```python
from build123d import *

# Parameters (mm, degrees)
BOSS_EXTRUDE1_DEPTH     = 100
BOSS_EXTRUDE1_TAPER     = 18.43
SKETCH2_W               = 170
SKETCH2_H               = 190
BOSS_EXTRUDE2_DEPTH     = 90
SKETCH3_R               = 1.35
BOSS_EXTRUDE3_DEPTH     = 10
SKETCH4_W               = 180
SKETCH4_H               = 50
CUT_EXTRUDE1_DEPTH      = 286.000000111
SKETCH5_R               = 2.5
CUT_EXTRUDE2_DEPTH      = 10
SKETCH6_R               = 8
CUT_EXTRUDE3_DEPTH      = 10
MIRROR4_COPY_1_SKETCH_R = 8
MIRROR4_COPY_1_DEPTH    = 10


with BuildPart() as part:
    # Sketch1 → Boss-Extrude1 (new body)
    with BuildSketch(Plane(origin=(0, 0, 0), x_dir=(1, 0, 0), z_dir=(0, 1, 0))):
        Polygon((-140, -45), (-125, -60), (-95, -90), (95, -90), (140, -45), (140, 45), (95, 90), (-95, 90), (-140, 45), align=None)
    extrude(amount=BOSS_EXTRUDE1_DEPTH, taper=BOSS_EXTRUDE1_TAPER)

    # Sketch2 → Boss-Extrude2 (add, symmetric)
    with BuildSketch(Plane.XY):
        with Locations((0, 45)):
            Rectangle(SKETCH2_W, SKETCH2_H)
    extrude(amount=BOSS_EXTRUDE2_DEPTH, both=True)

    # Sketch3 → Boss-Extrude3 (add, symmetric)
    with BuildSketch(Plane(origin=(0, 140, 0), x_dir=(1, 0, 0), z_dir=(0, 1, 0))):
        with Locations(Location((-70, 87.5, 0), (0, 0, 90))):
            Circle(SKETCH3_R)
        with Locations(Location((70, 87.5, 0), (0, 0, 90))):
            Circle(SKETCH3_R)
    boss_extrude3 = extrude(amount=BOSS_EXTRUDE3_DEPTH, both=True)

    # Mirror1: Boss-Extrude3 across plane
    add(boss_extrude3.mirror(Plane.XY))

    # Sketch4 → Cut-Extrude1 (cut, through all)
    with BuildSketch(Plane.ZY.offset(85)):
        with Locations((0, -25)):
            Rectangle(SKETCH4_W, SKETCH4_H)
    extrude(amount=-CUT_EXTRUDE1_DEPTH, mode=Mode.SUBTRACT)

    # Sketch5 → Cut-Extrude2 (cut)
    with BuildSketch(Plane(origin=(0, 0, -90), x_dir=(-1, 0, 0), z_dir=(0, 0, -1))):
        with Locations((-60, 133)):
            Circle(SKETCH5_R)
        with Locations((60, 133)):
            Circle(SKETCH5_R)
    cut_extrude2 = extrude(amount=-CUT_EXTRUDE2_DEPTH, mode=Mode.SUBTRACT)

    # Mirror2: Cut-Extrude2 across plane
    add(cut_extrude2.mirror(Plane.XY), mode=Mode.SUBTRACT)

    # Sketch6 → Cut-Extrude3 (cut)
    with BuildSketch(Plane(origin=(-83.254793164, 39.235386654, -83.254793164), x_dir=(-0.6068291050905237, 0.2859796255102721, 0.741602380665029), z_dir=(-0.6708397043943968, 0.31614582397380636, -0.6708397043943966))):
        with Locations(Location((23.427974197, -19.317213572, 0), (0, 0, 342.455867608))):
            Circle(SKETCH6_R)
        with Locations(Location((47.265100386, -26.853221472, 0), (0, 0, 342.455867608))):
            Circle(SKETCH6_R)
    cut_extrude3 = extrude(amount=-CUT_EXTRUDE3_DEPTH, mode=Mode.SUBTRACT)

    # Mirror3: Cut-Extrude3 across plane
    add(cut_extrude3.mirror(Plane.XY), mode=Mode.SUBTRACT)

    # Mirror4: Cut-Extrude3 across plane
    add(cut_extrude3.mirror(Plane(origin=(0, 0, 0), x_dir=(0, 0, 1), z_dir=(1, 0, 0))), mode=Mode.SUBTRACT)

    # Mirror4 copy 1 sketch → Mirror4 copy 1 (cut)
    with BuildSketch(Plane(origin=(83.254793164, 39.235386654, 83.254793164), x_dir=(0.6068291050905237, 0.2859796255102721, -0.741602380665029), z_dir=(0.6708397043943968, 0.31614582397380636, 0.6708397043943966))):
        with Locations(Location((23.427974197, -19.317213572, 0), (0, 0, 342.455867608))):
            Circle(MIRROR4_COPY_1_SKETCH_R)
        with Locations(Location((47.265100386, -26.853221472, 0), (0, 0, 342.455867608))):
            Circle(MIRROR4_COPY_1_SKETCH_R)
    extrude(amount=-MIRROR4_COPY_1_DEPTH, mode=Mode.SUBTRACT)


solid = part.part
```
Verification items for the finished model (mm, model axes). A direction names the side the tool comes from. Give positions to 0.01 mm unless a question says otherwise; leave off trailing zeros. Order: outer loops, then holes, each group sorted by start corner. A loop starts at its lowest first (then second) coordinate and runs counter-clockwise, first axis right, second up. Notation, with made-up numbers: M 10,-39.75 L 55,-39.75 A14 ccw 55,-12.75 Z; hole C -3.75,-0.5 d7. An arc over 180 degrees is marked long. Return JSON: item names as keys, results as strings. Group by question number.
1) Section check B-B on y = 118. Record the cut outline in (x, z), and give its area (3 significant figures).
2) Access from +Z, -Z, +X, -X, +Y, -Y to the whole of each face (thin tool, end or side, straight path). Record for faces 4 (the face through (-1, 71, 90)), 5 (the face through (-92, 100, 3)), 6 (the face through (-116.57, 25.41, -41.55)).
3) Go/stop test with flat-tipped pins: pin 1 Ø11 at (x, z) = (92.5, 20) entering from +Y; pin 2 Ø1.5 at (x, y) = (-59.5, 133) entering from +Z; pin 3 Ø1.5 at (y, z) = (32, -65.5) entering from -X. Record where each tip stops, or that it passes through.
4) Section check A-A on x = 16. Record the cut outline in (y, z).
5) Scan lines: line 1 (Y direction, x = 60, z = 85); line 2 (X direction, y = 133, z = 85.5); line 3 (Z direction, x = -117, y = 23). Record each from-to range of solid material in increasing order.
6) Mould release check, pull along Z, two halves, no side actions. Record for faces 1 (the face through (-1, 71, -90)), 2 (the face through (98.89, 25.41, 59.23)), 3 (the face through (-2, 0, -1)): pulls with the +Z half, pulls with the -Z half, needs draft (parallel to the pull), parting line crosses it, or undercut.
Answer block:
{
 "1": {"outline": "M -85,-90 L 85,-90 L 85,90 L -85,90 Z", "area": "30,600 mm^2"},
 "2": {"face 4": "+Z, +X, -X, +Y, -Y", "face 5": "+Z, -Z, -X, +Y", "face 6": "none"},
 "3": {"pin 1": "stops at y = 100", "pin 2": "stops at z = 80", "pin 3": "stops at x = -97.82"},
 "4": {"outline": "M 0,-90 L 140,-90 L 140,90 L 0,90 Z"},
 "5": {"line 1": "y = 0 to 130.5, 135.5 to 140", "line 2": "x = -85 to -62.5, -57.5 to 57.5, 62.5 to 85", "line 3": "z = -57.16 to -51.24, -42.25 to 42.25, 51.24 to 57.16"},
 "6": {"face 1": "pulls with the -Z half", "face 2": "undercut", "face 3": "needs draft"}
}
